Here's the drawing with two shaded views (mm, measured from the low corner). I have some questions. Give positions to 0.01 mm unless a question says otherwise; leave off trailing zeros. Write each loop counter-clockwise with the first axis right and the second up, starting at its lowest first coordinate (ties: lowest second). Pieces come first, ordered by that corner, then holes. Notation, with made-up numbers: (6, 21) - (58, 21) arc R9 cw to (58, 29) - close; hole circle Ø9 at (85.5, -21). An arc over 180 degrees is marked (long way). Answer as CSV lines item,"result". Start each with the question number.
Q1. If I drill on line 1 along X through (y, z) = (12, 19); line 2 along Z through (x, y) = (254, 12.25); line 3 along Y through (x, z) = (449.5, 12), over which ranges is the centre line in solid material (lowest first)?
Q2. Will these pins go through, and if not, where does the flat tip stop? pin 1 Ø9 at (x, z) = (254, 19.05) entering from -Y; pin 2 Ø1.5 at (x, y) = (374, 17) entering from -Z (1 decimal); pin 3 Ø1 at (x, z) = (296, 6) entering from +Y (1 decimal); pin 4 Ø2 at (x, z) = (465.5, 22.5) entering from -Y.
Q3. Imagine slicing it at B-B on x = 500. List the corners of the cut face in (y, z) for me, and give its area (3 significant figures).
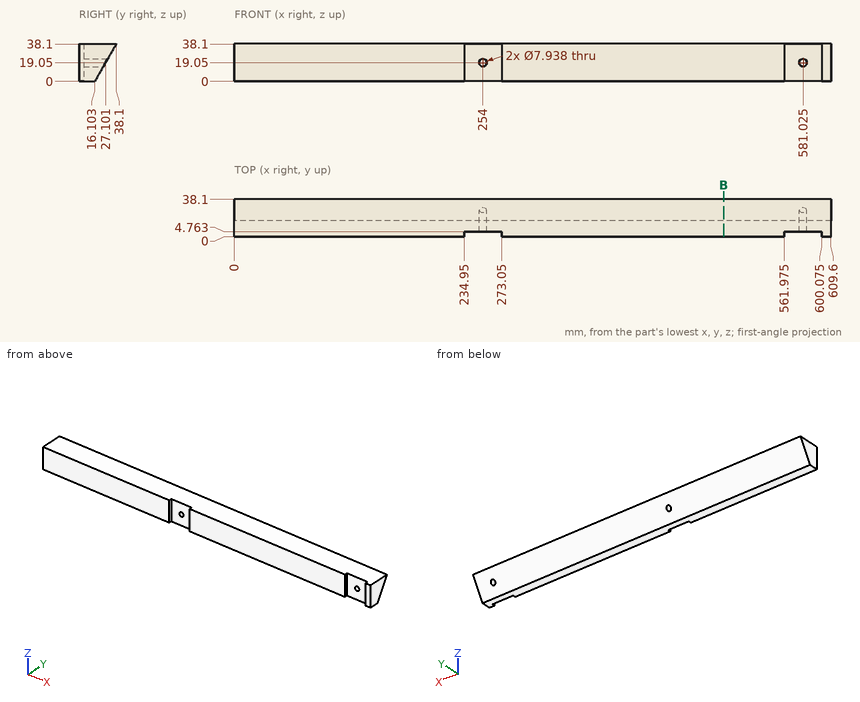
Conclusion:
1,line 1,"0 to 250.03, 257.97 to 577.06, 584.99 to 609.6"
1,line 2,"0 to 15.08, 23.02 to 38.1"
1,line 3,"0 to 23.03"
2,pin 1,"y = 4.76"
2,pin 2,"z = 0.3"
2,pin 3,"y = 19.9"
2,pin 4,"y = 0"
3,outline,"(0, 0) - (16.1, 0) - (38.1, 38.1) - (0, 38.1) - close"
3,area,"1,030 mm^2"
